CAD build for the part. Positions are in the model's coordinates, mm. A direction names the side the tool comes from. Coordinates: 2 decimals unless noted, no trailing zeros. Loops run counter-clockwise (first coordinate to the right, second up) from the corner with the lowest first, then second, coordinate; pieces in that order, holes last.
1) Wall check: line 1 along Y through (x, z) = (7, 3.5); line 2 along X through (y, z) = (1.75, 2.75); line 3 along Y through (x, z) = (6.5, -1.75). Give the ranges that are in metal, low to high.
2) Saw through at D-D, the plane x = 2. Write the cut outline in (y, z).
3) Pin check, flat tip, straight feed: pin 1 Ø0.5 at (x, y) = (1.5, 4) entering from +Z. Stop position of the tip, or through.
4) Saw through at B-B, the plane y = 1.23. Write the cut outline in (x, z).
5) Saw through at A-A, the plane z = 6.5. Write the cut outline in (x, y), and give its area (3 significant figures).
6) Which spindle directions (+Z, -Z, +X, -X, +Y, -Y) get a long thin tool onto all of the face, cutting with end or side? Do faces 1 (the flat face through (3.9, 2.5, 8.6)), 2 (the flat face through (3.1, 1, 5)), 3 (the flat face through (4, 3, 0)). Say none if no direction does.
7) Saw through at C-C, the plane x = 4. Write the cut outline in (y, z).
8) Two-plate mould, pull along Y, no slides. Class faces 4 (the flat face through (5.64, 4, 5)), 5 (the flat face through (8, 2, 4)): +Y half, -Y half, draft (parallel to the pull), parting line (faces both ways), or undercut.
Autodesk Fusion 360 part; units mm, degrees
sketch "スケッチ1" plane through (0, 0, 0) normal (0, 0, 1) x (1, 0, 0)
  line L0 (0, 0) -> (8, 0)
  line L1 (8, 0) -> (8, 5)
  line L2 (8, 5) -> (0, 5)
  line L3 (0, 5) -> (0, 0)
  circle A0 centre (1.46, 1.23) radius 0.25
  dimension "d1" = 8
  dimension "d2" = 5
  dimension "d15" = 0.5
  dimension "d16" = 1.23
  dimension "d17" = 1.46
extrude "押し出し1" add sketch "スケッチ1" along normal blind 8.6 contours L0 L1 L2 L3 | A0
sketch "スケッチ2" plane through (0, 0, 8.6) normal (0, 0, 1) x (-1, 0, 0)
  line L0 (0, -5) -> (0, 0)
  line L1 (0, 0) -> (-8, 0)
  line L2 (-8, 0) -> (-8, -5)
  line L3 (-8, -5) -> (0, -5)
  line L4 (-0.56, -0.33) -> (-2.36, -0.33)
  line L5 (-2.36, -0.33) -> (-2.36, -2.13)
  line L6 (-2.36, -2.13) -> (-0.56, -2.13)
  line L7 (-0.56, -2.13) -> (-0.56, -0.33)
  dimension "d5" = 1.8
  dimension "d6" = 1.8
  dimension "d7" = 0.33
  dimension "d8" = 0.56
extrude "押し出し2" cut sketch "スケッチ2" against normal blind 8 contours L4 L5 L6 L7
pattern_linear "R パターン1" count 3 spacing 2.54 along (1, 0, 0) count 2 spacing 2.54 along (0, 1, 0) of "押し出し2"
extrude "押し出し3" add sketch "スケッチ1" against normal blind 3 contours A0
pattern_linear "R パターン2" count 3 spacing 2.54 along (1, 0, 0) count 2 spacing 2.54 along (0, 1, 0) of "押し出し3"
Data:
1. line 1: y = 0 to 0.33, 2.13 to 2.87, 4.67 to 5
1. line 2: x = 0 to 0.56, 2.36 to 3.1, 4.9 to 5.64, 7.44 to 8
1. line 3: y = 0.98 to 1.48, 3.52 to 4.02
2. outline: (0, 0) - (5, 0) - (5, 8.6) - (4.67, 8.6) - (4.67, 0.6) - (2.87, 0.6) - (2.87, 8.6) - (2.13, 8.6) - (2.13, 0.6) - (0.33, 0.6) - (0.33, 8.6) - (0, 8.6) - close
3. pin 1: stops at z = 0.6
4. outline: (0, 0) - (1.21, 0) - (1.21, -3) - (1.71, -3) - (1.71, 0) - (3.75, 0) - (3.75, -3) - (4.25, -3) - (4.25, 0) - (6.29, 0) - (6.29, -3) - (6.79, -3) - (6.79, 0) - (8, 0) - (8, 8.6) - (7.44, 8.6) - (7.44, 0.6) - (5.64, 0.6) - (5.64, 8.6) - (4.9, 8.6) - (4.9, 0.6) - (3.1, 0.6) - (3.1, 8.6) - (2.36, 8.6) - (2.36, 0.6) - (0.56, 0.6) - (0.56, 8.6) - (0, 8.6) - close
5. outline: (0, 0) - (8, 0) - (8, 5) - (0, 5) - close; hole (0.56, 0.33) - (2.36, 0.33) - (2.36, 2.13) - (0.56, 2.13) - close; hole (0.56, 2.87) - (2.36, 2.87) - (2.36, 4.67) - (0.56, 4.67) - close; hole (3.1, 0.33) - (4.9, 0.33) - (4.9, 2.13) - (3.1, 2.13) - close; hole (3.1, 2.87) - (4.9, 2.87) - (4.9, 4.67) - (3.1, 4.67) - close; hole (5.64, 0.33) - (7.44, 0.33) - (7.44, 2.13) - (5.64, 2.13) - close; hole (5.64, 2.87) - (7.44, 2.87) - (7.44, 4.67) - (5.64, 4.67) - close
5. area: 20.6 mm2
6. face 1: +Z, +X, -X, +Y, -Y
6. face 2: +Z
6. face 3: -Z
7. outline: (0, 0) - (0.98, 0) - (0.98, -3) - (1.48, -3) - (1.48, 0) - (3.52, 0) - (3.52, -3) - (4.02, -3) - (4.02, 0) - (5, 0) - (5, 8.6) - (4.67, 8.6) - (4.67, 0.6) - (2.87, 0.6) - (2.87, 8.6) - (2.13, 8.6) - (2.13, 0.6) - (0.33, 0.6) - (0.33, 8.6) - (0, 8.6) - close
8. face 4: undercut
8. face 5: draft
